Input: part model. Units: mm. Frame: model coordinates. A direction names the side the tool comes from. Give positions to 0.01 mm unless a question says otherwise; leave off trailing zeros. Loops run counter-clockwise (first coordinate to the right, second up) from the corner with the lowest first, then second, coordinate; pieces in that order, holes last. Notation, with made-up numbers: (30, 5.25) - (77, 5.25) arc R24 ccw to (77, 43.25) - close; hole circle Ø7 at (87, 26). An arc over 180 degrees is marked (long way). Answer as a JSON object with one key per item and string values. Group by question number.
(1) Section query B-B (x = 6.5). Return loops of the section in (y, z), plus the area to 3 significant figures.
(2) Access query for faces 1 (the flat face through (6, 10, 29)), 2 (the cylindrical face through (5.741, 6.583, 11.465)). Directions: +Z, -Z, +X, -X, +Y, -Y. A direction counts if a zero-diameter tool reaches every point of the face in a straight line with its end or side. Return the directions, or none.
(3) Material intervals for L1, parallel to Z at x = 3.25, y = 2.5; L2, parallel to Z at x = 6.5, y = 6; L3, parallel to X at y = 8, z = 8.75, sorted ascending.
(4) Section query D-D (x = 10.5). Return loops of the section in (y, z), plus the area to 3 significant figures.
(5) Section query A-A (y = 10). Return loops of the section in (x, z), plus the area to 3 significant figures.
(6) Pin query (flat end, axial travel): P1, Ø2, axis at y = 10.5, z = 21, coming from the -X side; P2, Ø4, axis at x = 7, z = 18, coming from the +Y side; P3, Ø4, axis at x = 6, z = 13, coming from the -Y side. Return the tip coordinate at first contact, or that it passes through.
(7) Section query C-C (z = 7.5). Return loops of the section in (x, y), plus the area to 3 significant figures.
```python
from build123d import *

# Parameters (mm, degrees)
SKETCH022_W  = 13
SKETCH022_H  = 16.7
PAD020_DEPTH = 6
SKETCH023_R  = 4.5
PAD021_DEPTH = 3
SKETCH024_R  = 3.5
PAD022_DEPTH = 5
SKETCH025_R  = 3
PAD023_DEPTH = 15


with BuildPart() as part:
    # Sketch022 → Pad020 (new body)
    with BuildSketch(Plane.XY):
        with Locations((6.5, 8.35)):
            Rectangle(SKETCH022_W, SKETCH022_H)
    extrude(amount=PAD020_DEPTH)

    # Sketch023 (on Face6 of Pad020) → Pad021 (join)
    with BuildSketch(Plane.XY.offset(6)):
        with Locations((6.5, 10)):
            Circle(SKETCH023_R)
    extrude(amount=PAD021_DEPTH)

    # Sketch024 (on Face8 of Pad021) → Pad022 (join)
    with BuildSketch(Plane.XY.offset(9)):
        with Locations((6.5, 10)):
            Circle(SKETCH024_R)
    extrude(amount=PAD022_DEPTH)

    # Sketch025 (on Face10 of Pad022) → Pad023 (join)
    with BuildSketch(Plane.XY.offset(14)):
        with Locations((6.5, 10)):
            Circle(SKETCH025_R)
    extrude(amount=PAD023_DEPTH)


solid = part.part
```
Recorded:
{
 "1": {"outline": "(0, 0) - (16.7, 0) - (16.7, 6) - (14.5, 6) - (14.5, 9) - (13.5, 9) - (13.5, 14) - (13, 14) - (13, 29) - (7, 29) - (7, 14) - (6.5, 14) - (6.5, 9) - (5.5, 9) - (5.5, 6) - (0, 6) - close", "area": "252 mm^2"},
 "2": {"face 1": "+Z, +X, -X, +Y, -Y", "face 2": "+Z"},
 "3": {"L1": "z = 0 to 6", "L2": "z = 0 to 9", "L3": "x = 2.47 to 10.53"},
 "4": {"outline": "(0, 0) - (16.7, 0) - (16.7, 6) - (12.06, 6) - (12.06, 9) - (7.94, 9) - (7.94, 6) - (0, 6) - close", "area": "113 mm^2"},
 "5": {"outline": "(0, 0) - (13, 0) - (13, 6) - (11, 6) - (11, 9) - (10, 9) - (10, 14) - (9.5, 14) - (9.5, 29) - (3.5, 29) - (3.5, 14) - (3, 14) - (3, 9) - (2, 9) - (2, 6) - (0, 6) - close", "area": "230 mm^2"},
 "6": {"P1": "stops at x = 3.5", "P2": "stops at y = 13", "P3": "stops at y = 6.5"},
 "7": {"outline": "circle Ø9 at (6.5, 10)", "area": "63.6 mm^2"}
}
